from build123d import *

# Parameters (mm, degrees)
SKETCH3_R           = 1.9
SKETCH3_R_2         = 1.2
BOSS_EXTRUDE4_DEPTH = 3.5
SKETCH3_3_R         = 5.9
SKETCH3_3_R_2       = 4.9
BOSS_EXTRUDE5_DEPTH = 2
BOSS_EXTRUDE6_DEPTH = 0.25
CIRPATTERN1_COUNT   = 3


with BuildPart() as part:
    # Sketch3 → Boss-Extrude4 (new body)
    with BuildSketch(Plane.XY):
        Circle(SKETCH3_R)
        Circle(SKETCH3_R_2, mode=Mode.SUBTRACT)
    extrude(amount=-BOSS_EXTRUDE4_DEPTH)



with BuildPart() as body_2:
    # Sketch3<3> → Boss-Extrude5 (new body)
    with BuildSketch(Plane.XY):
        Circle(SKETCH3_3_R)
        Circle(SKETCH3_3_R_2, mode=Mode.SUBTRACT)
    extrude(amount=-BOSS_EXTRUDE5_DEPTH)


with BuildPart() as part_1:
    add(part.part)

    add(body_2.part)  # Boss-Extrude6 merges body 2
    # Sketch5 → Boss-Extrude6 (add, symmetric)
    with BuildSketch(Plane(origin=(0, 0, 0), x_dir=(0, 0, -1), z_dir=(1, 0, 0))):
        Polygon((0, 4.9), (0, 1.903401583), (0, 1.703401583), (3.5, 1.703401583), (3.5, 1.903401583), (2, 4.9), align=None)
    boss_extrude6 = extrude(amount=BOSS_EXTRUDE6_DEPTH, both=True)

    # CirPattern1: Boss-Extrude6 ×3 about axis
    cirpattern1_axis = Axis((0, 0, 0), (0, 0, 1))
    for i in range(1, CIRPATTERN1_COUNT):
        add(boss_extrude6.rotate(cirpattern1_axis, i * 360 / CIRPATTERN1_COUNT))


solid = part_1.part
Design review of the part built by this model. Coordinates are the model's own, in mm. A direction names the side the tool comes from. Coordinates: 2 decimals unless noted, no trailing zeros. Order: outer loops, then holes, each group sorted by start corner. A loop starts at its lowest first (then second) coordinate and runs counter-clockwise, first axis right, second up.
Item 1: Take a section at C-C, the plane z = -2.8. Write out the cut boundary in (x, y), then the cut area to 3 significant figures.
Item 2: Take a section at A-A, the plane y = 0. Write out the cut boundary in (x, z), then the cut area to 3 significant figures.
Item 3: For pin 1 Ø1.5 at (y, z) = (3.5, -1.5) entering from +X; pin 2 Ø3 at (x, y) = (-3.5, 2) entering from -Z; pin 3 Ø2 at (x, y) = (0, 0) entering from -Z; pin 4 Ø1.5 at (y, z) = (3.5, -1) entering from -X, all flat-tipped, find the tip position at first contact; note any pin that passes through.
Item 4: The part is to be moulded in two halves that separate along Y. For faces 1 (the flat face through (2.93, -1.69, -2.76)), 2 (the cylindrical face through (-1.633, 0.971, -1.726)), 3 (the flat face through (1, -1, 0)), say which applies: pulls with the +Y half, pulls with the -Y half, needs draft (parallel to the pull), parting line crosses it, or undercut.
Item 5: For faces 4 (the flat face through (0, 3.38, -2.76)), 5 (the cylindrical face through (1.657, 0.929, -1.726)), 6 (the flat face through (1, 5, -2)), list the 3-axis set-ups (+Z, -Z, +X, -X, +Y, -Y) from which the entire face can be reached by the end or side of a thin tool; tool diameter is ignored.
Item 6: Take a section at D-D, the plane y = 2.5. Write out the cut boundary in (x, z), then the cut area to 3 significant figures.
Item 7: Take a section at B-B, the plane x = 0. Write out the cut boundary in (y, z), then the cut area to 3 significant figures.
Item 8: For line 1 (Y direction, x = 0, z = -0.9); line 2 (Y direction, x = 3, z = -0.2); line 3 (X direction, y = -1, z = -1), list the stretches that pass through material, from the lowest coordinate up.
The answers:
1. outline: (-2.98, -1.43) - (-2.73, -1.87) - (-1.51, -1.16) arc R1.9 ccw to (1.51, -1.16) - (2.73, -1.87) - (2.98, -1.43) - (1.76, -0.73) arc R1.9 ccw to (0.25, 1.88) - (0.25, 3.3) - (-0.25, 3.3) - (-0.25, 1.88) arc R1.9 ccw to (-1.76, -0.73) - close; hole circle Ø2.4 at (0, 0)
1. area: 8.93 mm2
2. outline: (-5.9, -2) - (-4.9, -2) - (-4.9, 0) - (-5.9, 0) - close; (-1.9, -3.5) - (-1.2, -3.5) - (-1.2, 0) - (-1.9, 0) - close; (1.2, -3.5) - (1.9, -3.5) - (1.9, 0) - (1.2, 0) - close; (4.9, -2) - (5.9, -2) - (5.9, 0) - (4.9, 0) - close
2. area: 8.90 mm2
3. pin 1: stops at x = 5.22
3. pin 2: stops at z = -2
3. pin 3: passes through
3. pin 4: stops at x = -5.22
4. face 1: pulls with the -Y half
4. face 2: undercut
4. face 3: needs draft
5. face 4: -Z, +X, -X, +Y
5. face 5: +Z, -Z
5. face 6: -Z
6. outline: (-5.34, -2) - (-4.21, -2) - (-4.21, 0) - (-5.34, 0) - close; (-0.25, -3.2) - (0.25, -3.2) - (0.25, 0) - (-0.25, 0) - close; (4.21, -2) - (5.34, -2) - (5.34, 0) - (4.21, 0) - close
6. area: 6.12 mm2
7. outline: (-5.9, -2) - (-4.9, -2) - (-4.9, 0) - (-5.9, 0) - close; (-1.9, -3.5) - (-1.2, -3.5) - (-1.2, 0) - (-1.9, 0) - close; (1.2, -3.5) - (1.9, -3.5) - (4.9, -2) - (5.9, -2) - (5.9, 0) - (1.2, 0) - close
7. area: 17.2 mm2
8. line 1: y = -5.9 to -4.9, -1.9 to -1.2, 1.2 to 5.9
8. line 2: y = -5.08 to -3.87, -2.02 to -1.44, 3.87 to 5.08
8. line 3: x = -5.81 to -4.8, -2.23 to -0.66, 0.66 to 2.23, 4.8 to 5.81
